```python
from build123d import *

# Parameters (mm, degrees)
ESQUISSE1_R             = 20
BOSS_EXTRU_1_DEPTH      = 10
ESQUISSE2_R             = 4
ENL_V_MAT_EXTRU_1_DEPTH = 11
ESQUISSE3_R             = 5
ENL_V_MAT_EXTRU_2_DEPTH = 5
ESQUISSE4_R             = 12
BOSS_EXTRU_2_DEPTH      = 5
ESQUISSE5_R             = 4
ENL_V_MAT_EXTRU_6_DEPTH = 16


with BuildPart() as part:
    # Esquisse1 → Boss.-Extru.1 (new body)
    with BuildSketch(Plane.XY):
        with Locations((0, 280)):
            Circle(ESQUISSE1_R)
    extrude(amount=BOSS_EXTRU_1_DEPTH)

    # Esquisse2 → Enlèv. mat.-Extru.1 (cut, through all)
    with BuildSketch(Plane.XY.offset(10)):
        with Locations((0, 280)):
            Circle(ESQUISSE2_R)
    extrude(amount=-ENL_V_MAT_EXTRU_1_DEPTH, mode=Mode.SUBTRACT)

    # Esquisse3 → Enlèv. mat.-Extru.2 (cut)
    with BuildSketch(Plane.XY.offset(10)):
        with Locations((0, 280)):
            Circle(ESQUISSE3_R)
    extrude(amount=-ENL_V_MAT_EXTRU_2_DEPTH, mode=Mode.SUBTRACT)

    # Esquisse4 → Boss.-Extru.2 (add)
    with BuildSketch(Plane(origin=(0, 0, 0), x_dir=(-1, 0, 0), z_dir=(0, 0, -1))):
        with Locations(Location((0, 280, 0), (0, 0, 180))):  # turned: the seam where the file's is
            Circle(ESQUISSE4_R)
    extrude(amount=BOSS_EXTRU_2_DEPTH)

    # Esquisse5 → Enlèv. mat.-Extru.6 (cut, through all)
    with BuildSketch(Plane(origin=(0, 0, -5), x_dir=(-1, 0, 0), z_dir=(0, 0, -1))):
        with Locations(Location((0, 280, 0), (0, 0, 180))):  # turned: the seam where the file's is
            Circle(ESQUISSE5_R)
    extrude(amount=-ENL_V_MAT_EXTRU_6_DEPTH, mode=Mode.SUBTRACT)


solid = part.part
```
Design review of the part built by this model. Coordinates are the model's own, in mm. A direction names the side the tool comes from. Give positions to 0.01 mm unless a question says otherwise; leave off trailing zeros. Order: outer loops, then holes, each group sorted by start corner. A loop starts at its lowest first (then second) coordinate and runs counter-clockwise, first axis right, second up. Notation, with made-up numbers: (26.25, 85) -> (39.25, 85) arc R15 cw to (39.25, 95) -> close; hole circle Ø10 at (-8.5, 25.5). An arc over 180 degrees is marked (long way). Write each question's results on one line, items separated by ' | '. Start each with the question number.
Q1. Machinability: for faces 1 (the flat face through (9, 271, 0)), 2 (the cylindrical face through (-0.651, 284.957, 7.535)), 3 (the flat face through (-3, 277, -5)), which of the approach directions +Z, -Z, +X, -X, +Y, -Y give a long, thin tool a straight path to every point of the face, cutting with its end or side? Answer none if there is none.
Q2. Add section C-C on z = 6.25. Give the boundary of the cut face in (x, y), and give its area (3 significant figures).
Q3. Mouldability with a two-part tool opening along Y and no side actions: class faces 4 (the flat face through (4, 276, 10)), 5 (the cylindrical face through (-2.601, 291.715, -2.465)), 6 (the cylindrical face through (1.846, 283.549, -0.07)) as +Y half, -Y half, draft (parallel to the pull), parting line (faces both ways), or undercut.
Q4. Add section A-A on x = 0. Give the boundary of the cut face in (y, z), and give its area (3 significant figures).
Q5. Add section D-D on x = 10.5. Give the boundary of the cut face in (y, z).
Q6. Add section B-B on y = 280. Give the boundary of the cut face in (x, z), and give its area (3 significant figures).
Q7. For pin 1 (1.5 mm diameter, centred on y = 264, z = 5, fed in from -X); pin 2 (2 mm diameter, centred on y = 268, z = 6, fed in from +X); pin 3 (6.5 mm diameter, centred on x = 0, y = 280, fed in from -Z); pin 4 (1 mm diameter, centred on x = -9.5, z = 4, fed in from +Y), all flat-tipped, find the tip position at first contact; note any pin that passes through.
Q8. Wall thickness on L1, parallel to Y at x = 0, z = 8.65; L2, parallel to Y at x = 0, z = -2.25; L3, parallel to Z at x = -16, y = 290.5: over which ranges is each line inside the solid? List them lowest first. Write a range as from..to.
Found:
1) face 1: -Z | face 2: +Z | face 3: -Z, +X, -X, +Y, -Y
2) outline: circle Ø40 at (0, 280); hole circle Ø10 at (0, 280) | area: 1,180 mm2
3) face 4: draft | face 5: parting line | face 6: undercut
4) outline: (260, 0) -> (268, 0) -> (268, -5) -> (276, -5) -> (276, 5) -> (275, 5) -> (275, 10) -> (260, 10) -> close; (284, -5) -> (292, -5) -> (292, 0) -> (300, 0) -> (300, 10) -> (285, 10) -> (285, 5) -> (284, 5) -> close | area: 390 mm2
5) outline: (262.98, 0) -> (274.19, 0) -> (274.19, -5) -> (285.81, -5) -> (285.81, 0) -> (297.02, 0) -> (297.02, 10) -> (262.98, 10) -> close
6) outline: (-20, 0) -> (-12, 0) -> (-12, -5) -> (-4, -5) -> (-4, 5) -> (-5, 5) -> (-5, 10) -> (-20, 10) -> close; (4, -5) -> (12, -5) -> (12, 0) -> (20, 0) -> (20, 10) -> (5, 10) -> (5, 5) -> (4, 5) -> close | area: 390 mm2
7) pin 1: stops at x = -12.94 | pin 2: stops at x = 16.7 | pin 3: passes through | pin 4: stops at y = 297.86
8) L1: y = 260..275, 285..300 | L2: y = 268..276, 284..292 | L3: z = 0..10
